Design review of the part built by this model. Coordinates are the model's own, in mm. Coordinates: 2 decimals unless noted, no trailing zeros. Write each loop counter-clockwise with the first axis right and the second up, starting at its lowest first coordinate (ties: lowest second). Pieces come first, ordered by that corner, then holes. Notation, with made-up numbers: (89.25, -18.5) -> (97.25, -18.5) arc R19 ccw to (97.25, 7.5) -> close; hole circle Ø4 at (61, 88). An arc over 180 degrees is marked (long way). One line per question, with ' | ' between items. Start each with the question number.
Q1. Add section A-A on y = -41.5. State the section outline as (x, z) points (3 decimals), and give its area (3 significant figures).
Q2. Wall thickness on probe 1 along Z at (x, y) = (87.5, -45); probe 2 along Z at (x, y) = (111.5, -41); probe 3 along Y at (x, z) = (88.5, 31.5): over which ranges is each line inside the solid? List them lowest first.
Q3. Add section B-B on x = 98. State the section outline as (y, z) points.
Q4. Add section D-D on z = 31. State the section outline as (x, y) points (3 decimals).
Q5. For P1, Ø6, axis at y = -24, z = 27.5, coming from the -X side (3 decimals); P2, Ø1, axis at x = 113.5, z = 13, coming from the -Y side; P3, Ø3, axis at x = 98.5, z = 31, coming from the +Y side; P4, Ø20.5, axis at x = 104.5, y = -19, coming from the +Z side, all flat-tipped, find the tip position at first contact; note any pin that passes through.
Q6. Add section C-C on y = -14. State the section outline as (x, z) points (3 decimals).
Autodesk Inventor part; units mm, degrees
ref_plane "Work Plane1" through (85.725, 80.736, -75.2679) normal (-1, 0, 0) x (0, -0.7045, -0.7097)
ref_plane "YZ Plane" through (0, 0, 0) normal (1, 0, 0) x (0, 1, 0)
ref_plane "XZ Plane" through (0, 0, 0) normal (0, 1, 0) x (-1, 0, 0)
ref_plane "Work Plane1" through (85.725, 80.736, -75.2679) normal (-1, 0, 0) x (0, -0.7045, -0.7097)
sketch "Sketch1" plane through (85.725, 80.736, -75.2679) normal (-1, 0, 0) x (0, -0.7045, -0.7097)
  line L0 (3.4608, 0) -> (3.4607, 241.3)
  line L1 (5.6975, 112.5782) -> (38.7126, 145.837)
  line L2 (3.4608, 110.3249) -> (5.6975, 112.5782)
  line L3 (38.7126, 145.837) -> (36.4593, 148.0738)
  line L4 (36.4593, 148.0738) -> (6.6358, 118.0301)
  line L5 (6.6358, 118.0301) -> (6.6358, 177.6787)
  line L6 (6.6358, 177.6787) -> (3.4607, 177.6787)
  line L7 (3.4607, 177.6787) -> (3.4608, 110.3249)
  line L8 (3.4608, 110.3249) -> (38.7126, 145.837)
  dimension "d0" = 3.175
  dimension "d1" = 3.175
extrude "Extrusion1" add sketch "Sketch1" against normal blind 41.275
properties part number "Support"
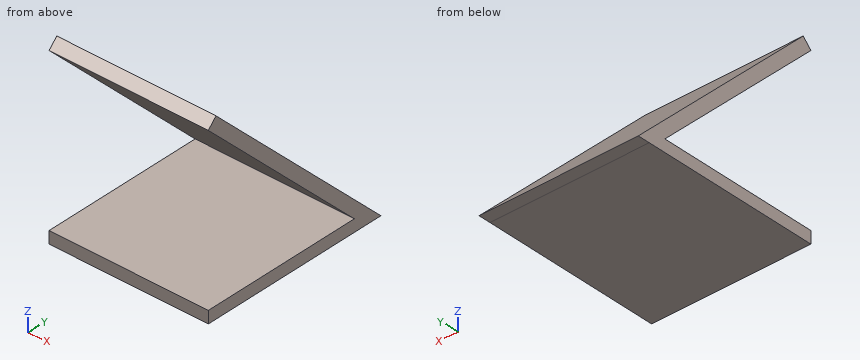
Output values:
1) outline: (85.725, 0) -> (127, 0) -> (127, 3.175) -> (85.725, 3.175) -> close; (85.725, 36.722) -> (127, 36.722) -> (127, 41.196) -> (85.725, 41.196) -> close | area: 316 mm2
2) probe 1: z = 0 to 3.18, 40.2 to 44.67 | probe 2: z = 0 to 3.18, 36.23 to 40.7 | probe 3: y = -36.24 to -31.73
3) outline: (-50.04, 0) -> (-3.17, 0) -> (0, 0) -> (-47.8, 47.45) -> (-50.04, 45.2) -> (-7.71, 3.18) -> (-50.04, 3.18) -> close
4) outline: (85.725, -35.735) -> (127, -35.735) -> (127, -31.229) -> (85.725, -31.229) -> close
5) P1: stops at x = 85.725 | P2: stops at y = -18.11 | P3: stops at y = -29.72 | P4: stops at z = 29.04
6) outline: (85.725, 0) -> (127, 0) -> (127, 3.175) -> (85.725, 3.175) -> close; (85.725, 9.424) -> (127, 9.424) -> (127, 13.898) -> (85.725, 13.898) -> close
